```python
from build123d import *

# Parameters (mm, degrees)
BOX019_W               = 127
BOX019_H               = 10.668
BOX019_DEPTH           = 30
BOX019_PLACEMENT_ANGLE = 97.5889000001
BOX018_W               = 609.6
BOX018_H               = 10.668
BOX018_DEPTH           = 60
BOX018_PLACEMENT_ANGLE = 97.5889000001


with BuildPart() as screensupporthole:
    # Box019 → Box019 (new body)
    with BuildSketch(Plane.XY):
        with Locations((63.5, 5.334)):
            Rectangle(BOX019_W, BOX019_H)
    extrude(amount=BOX019_DEPTH)


with BuildPart() as screensupporthole_1:
    # Box019 placement: moved
    add(screensupporthole.part.moved(Location((241.3, 462.432, 1143.32))).rotate(Axis((241.3, 462.432, 1143.32), (1, 0, 0)), BOX019_PLACEMENT_ANGLE))


with BuildPart() as screenbottom:
    # Box018 → Box018 (new body)
    with BuildSketch(Plane.XY):
        with Locations((304.8, 5.334)):
            Rectangle(BOX018_W, BOX018_H)
    extrude(amount=BOX018_DEPTH)


with BuildPart() as screenbottom_1:
    # Box018 placement: moved
    add(screenbottom.part.moved(Location((10.668, 462.432, 1143.32))).rotate(Axis((10.668, 462.432, 1143.32), (1, 0, 0)), BOX018_PLACEMENT_ANGLE))

    # Cut003: cut ScreenSupportHole
    add(screensupporthole_1.part, mode=Mode.SUBTRACT)


solid = screenbottom_1.part
```
Here's how the part is built. I have some questions about the finished solid (model axes, mm). A direction names the side the tool comes from. Round coordinates to 2 decimals unless told otherwise and drop trailing zeros. Write each loop counter-clockwise with the first axis right and the second up, starting at its lowest first coordinate (ties: lowest second). Pieces come first, ordered by that corner, then holes.
Q1. Please list where these lines run through material, in increasing order: probe 1 along X at (y, z) = (456.5, 1150); probe 2 along Z at (x, y) = (231.5, 432); probe 3 along Y at (x, z) = (242, 1143).
Q2. If we section it at A-A on y = 455.5: Write out the boundary of the cut face in (x, z), plus the area to 3 significant figures.
Q3. If we section it at C-C on y = 422.5: Write out the boundary of the cut face in (x, z).
Q4. If we section it at B-B on x = 60.5: Write out the boundary of the cut face in (y, z).
Q5. Will these pins go through, and if not, where does the flat tip stop? P1, Ø1.5, axis at x = 215.5, y = 436, coming from the +Z side; P2, Ø1.5, axis at x = 176.5, y = 422, coming from the +Z side; P3, Ø3, axis at x = 311.5, z = 1141, coming from the -Y side.
Q6. Which directions (+Z, -Z, +X, -X, +Y, -Y) give clear straight access to the entire face, cutting with the end or side of a thin tool? Please do faces 1 (the flat face through (303.91, 431.98, 1144.72)), 2 (the flat face through (311.201, 425.094, 1149.108)).
Q7. If we mould it in two halves opening along X, with no side actions, what happens to faces 3 (the flat face through (368.3, 447, 1147)), 4 (the flat face through (620.268, 432, 1145)), 5 (the flat face through (311.201, 426.503, 1138.533)), 6 (the flat face through (241.3, 447, 1147))? For each: +X half, -X half, draft (parallel to the pull), parting line (faces both ways), or undercut.
Answer below:
1. probe 1: x = 10.67 to 241.3, 368.3 to 620.27
1. probe 2: z = 1139.27 to 1150.03
1. probe 3: y = 401.94 to 432.21
2. outline: (10.67, 1142.4) - (241.3, 1142.4) - (241.3, 1153.16) - (10.67, 1153.16) - close; (368.3, 1142.4) - (620.27, 1142.4) - (620.27, 1153.16) - (368.3, 1153.16) - close
2. area: 5,190 mm2
3. outline: (10.67, 1138) - (620.27, 1138) - (620.27, 1148.76) - (10.67, 1148.76) - close
4. outline: (401.55, 1145.97) - (402.96, 1135.4) - (462.43, 1143.32) - (461.02, 1153.89) - close
5. P1: stops at z = 1150.66
5. P2: stops at z = 1148.8
5. P3: stops at y = 402.01
6. face 1: +Z, +Y
6. face 2: +Z, +X, -X, -Y
7. face 3: undercut
7. face 4: +X half
7. face 5: draft
7. face 6: undercut
